```python
from build123d import *

# Parameters (mm, degrees)
SKETCH2_W           = 3.02065634
SKETCH2_H           = 7.518324789
CUT_EXTRUDE1_DEPTH  = 10
SKETCH3_W           = 0.5
SKETCH3_H           = 0.5
BOSS_EXTRUDE1_DEPTH = 27.5
SKETCH4_W           = 5.267687
SKETCH4_H           = 3.125919431
CUT_EXTRUDE2_DEPTH  = 13.75


with BuildPart() as part:
    # Sketch1 → Revolve1 (revolve)
    with BuildSketch(Plane.XY):
        with BuildLine():
            Line((0, 0), (3, 0))
            Line((3, 0), (3, 1.05))
            Line((3, 1.05), (2.5, 1.05))
            Line((2.5, 1.05), (2.5, 6.21))
            ThreePointArc((2.5, 6.21), (1.767766953, 7.977766953), (0, 8.71))
            Line((0, 8.71), (0, 6.21))
            Line((0, 6.21), (0, 0))
        make_face()
    revolve(axis=Axis((0, 6.21, 0), (0, -1, 0)))

    # Sketch2 → Cut-Extrude1 (cut)
    with BuildSketch(Plane.XZ):
        with Locations((-4.06032817, -1.07166668)):
            Rectangle(SKETCH2_W, SKETCH2_H)
    extrude(amount=-CUT_EXTRUDE1_DEPTH, mode=Mode.SUBTRACT)

    # Sketch3 → Boss-Extrude1 (add)
    with BuildSketch(Plane.XZ):
        with Locations((-1.5, 0)):
            Rectangle(SKETCH3_W, SKETCH3_H)
        with Locations((1.5, 0)):
            Rectangle(SKETCH3_W, SKETCH3_H)
    extrude(amount=BOSS_EXTRUDE1_DEPTH)

    # Sketch4 → Cut-Extrude2 (cut, symmetric)
    with BuildSketch(Plane.XY):
        with Locations((-2.6338435, -28.062959715)):
            Rectangle(SKETCH4_W, SKETCH4_H)
    extrude(amount=CUT_EXTRUDE2_DEPTH, both=True, mode=Mode.SUBTRACT)


solid = part.part
```
Here's how the part is built. I have some questions about the finished solid (model axes, mm). A direction names the side the tool comes from. Give positions to 0.01 mm unless a question says otherwise; leave off trailing zeros. Loops run counter-clockwise (first coordinate to the right, second up) from the corner with the lowest first, then second, coordinate; pieces in that order, holes last. Notation, with made-up numbers: (-34.5, 14.25) -> (-24.5, 14.25) arc R34 cw to (-24.5, 50.25) -> close; hole circle Ø5 at (72, -19.5). An arc over 180 degrees is marked (long way). Use one line per item in the form item = value. Start each with the question number.
1) For P1, Ø3, axis at x = 1.5, y = 2, coming from the +Z side; P2, Ø0.6, axis at x = -1.5, y = -16, coming from the +Z side; P3, Ø1.5, axis at x = 2, z = 1, coming from the -Y side, each with a flat end and sliding along its axis, tell me the tip position at first contact or that it passes through.
2) Imagine slicing it at D-D (y = 4). Please give me the cut outline in (x, z).
3) Which directions (+Z, -Z, +X, -X, +Y, -Y) give clear straight access to the entire face, cutting with the end or side of a thin tool? Please do faces 1 (the face through (-2.55, 0.5, 0)), 2 (the face through (2, 1.05, -2)).
4) Imagine slicing it at A-A (y = -18.5). Please give me the cut outline in (x, z).
5) Imagine slicing it at C-C (z = 1). Please give me the cut outline in (x, y).
6) Imagine slicing it at B-B (x = 0). Please give me the cut outline in (y, z), then the cut area to 3 significant figures.
7) Please list where these lines run through material, in increasing order: line 1 along X through (y, z) = (-22, 0); line 2 along Y through (x, z) = (2.55, 1.25); line 3 along Z through (x, y) = (1.55, -10.5).
Check values:
q1.P1 = 2.98
q1.P2 = 0.25
q1.P3 = 0
q2.outline = circle Ø5 at (0, 0)
q3.face_1 = +Z, -Z, -X, +Y, -Y
q3.face_2 = +Y
q4.outline = (-1.75, -0.25) -> (-1.25, -0.25) -> (-1.25, 0.25) -> (-1.75, 0.25) -> close; (1.25, -0.25) -> (1.75, -0.25) -> (1.75, 0.25) -> (1.25, 0.25) -> close
q5.outline = (-2.55, 0) -> (2.83, 0) -> (2.83, 1.05) -> (2.29, 1.05) -> (2.29, 6.21) arc R2.29 ccw to (-2.29, 6.21) -> (-2.29, 1.05) -> (-2.55, 1.05) -> close
q6.outline = (0, -3) -> (1.05, -3) -> (1.05, -2.5) -> (6.21, -2.5) arc R2.5 ccw to (6.21, 2.5) -> (1.05, 2.5) -> (1.05, 3) -> (0, 3) -> close
q6.area = 41.9 mm^2
q7.line_1 = -1.75 to -1.25, 1.25 to 1.75
q7.line_2 = 0 to 1.05
q7.line_3 = -0.25 to 0.25
